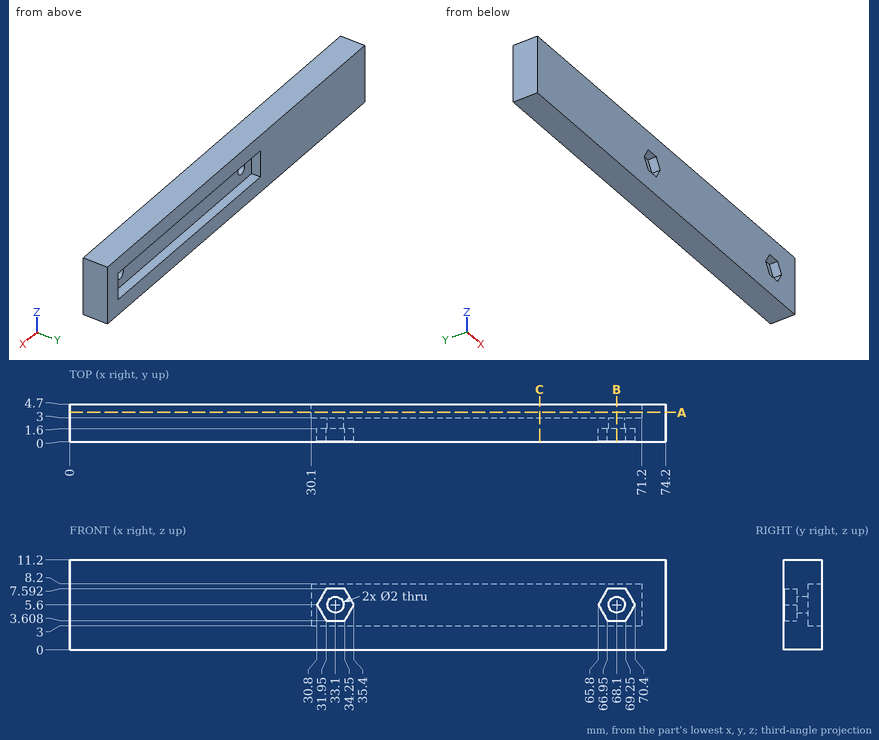
Drawing for the job (mm, zero at the part's lowest x, y, z). Coordinates: 2 decimals unless noted, no trailing zeros. Write each loop counter-clockwise with the first axis right and the second up, starting at its lowest first coordinate (ties: lowest second). Pieces come first, ordered by that corner, then holes. Notation, with made-up numbers: (72, 23.5) -> (110, 23.5) arc R16 ccw to (110, 27.5) -> close; hole circle Ø6 at (-17, -16). An arc over 180 degrees is marked (long way). One line per item, written item: value. Start each with the question number.
1) Slice it at C-C on x = 58.5. Write the cut outline in (y, z).
2) Flat gauge pins, fed straight in: pin 1 Ø1.5 at (x, y) = (11.5, 1) entering from -Z; pin 2 Ø1.8 at (x, z) = (68.1, 5.6) entering from +Y; pin 3 Ø2.5 at (x, z) = (59, 5.5) entering from +Y. Where does each tip first touch, or does it go through?
3) Slice it at B-B on x = 68.1. Write the cut outline in (y, z).
4) Probe probe 1 along X at (y, z) = (2.2, 5.6); probe 2 along Z at (x, y) = (68.1, 2.7); probe 3 along Z at (x, y) = (30.5, 4.4). List the from-to ranges inside material, lowest first.
5) Slice it at A-A on y = 3.65. Write the cut outline in (x, z), then the cut area to 3 significant figures.
Answers follow:
1. outline: (0, 0) -> (4.7, 0) -> (4.7, 3) -> (3, 3) -> (3, 8.2) -> (4.7, 8.2) -> (4.7, 11.2) -> (0, 11.2) -> close
2. pin 1: z = 0
2. pin 2: through
2. pin 3: y = 3
3. outline: (0, 0) -> (4.7, 0) -> (4.7, 3) -> (3, 3) -> (3, 4.6) -> (1.6, 4.6) -> (1.6, 3.61) -> (0, 3.61) -> close; (0, 7.59) -> (1.6, 7.59) -> (1.6, 6.6) -> (3, 6.6) -> (3, 8.2) -> (4.7, 8.2) -> (4.7, 11.2) -> (0, 11.2) -> close
4. probe 1: 0 to 32.1, 34.1 to 67.1, 69.1 to 74.2
4. probe 2: 0 to 4.6, 6.6 to 11.2
4. probe 3: 0 to 3, 8.2 to 11.2
5. outline: (0, 0) -> (74.2, 0) -> (74.2, 11.2) -> (0, 11.2) -> close; hole (30.1, 3) -> (71.2, 3) -> (71.2, 8.2) -> (30.1, 8.2) -> close
5. area: 617 mm2
